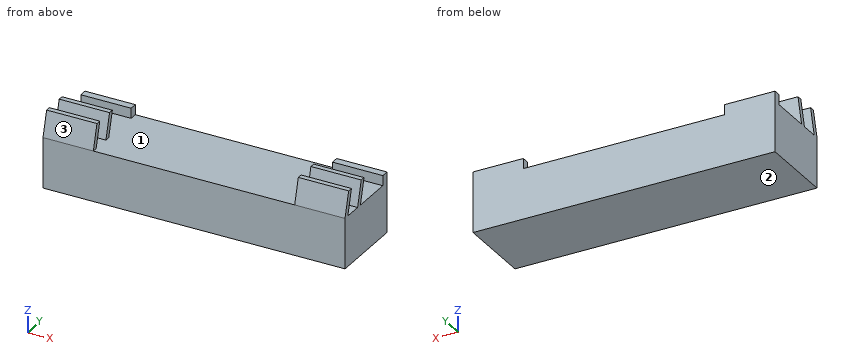
from build123d import *

# Parameters (mm, degrees)
F0_W     = 60
F0_H     = 15
F1_DEPTH = 10
F2_W     = 1.5
F2_H     = 2
F3_DEPTH = 10


with BuildPart() as f1:
    # F0 (on Top) → F1 (new body)
    with BuildSketch(Plane.XY):
        Rectangle(F0_W, F0_H)
    extrude(amount=F1_DEPTH)

    # F2 (on face) → F3 (join)
    with BuildSketch(Plane.YZ.offset(30)):
        Polygon((-6.205905, 14.829629), (-7.5, 10), (-6.5, 10), (-5.205905, 14.829629), align=None)
        Polygon((-3, 10), (-2, 10), (-0.705905, 14.829629), (-1.705905, 14.829629), align=None)
        with Locations((6.75, 11)):
            Rectangle(F2_W, F2_H)
    extrude(amount=-F3_DEPTH)

    # F4: F1 across plane


with BuildPart() as f1_1:
    add(f1.part)
    add(f1.part.mirror(Plane.YZ))


solid = f1_1.part
The model under review builds one solid part; all positions refer to its coordinate system, in mm. Face numbers are marked on the shaded views. Round coordinates to 2 decimals unless told otherwise and drop trailing zeros. Loops run counter-clockwise (first coordinate to the right, second up) from the corner with the lowest first, then second, coordinate; pieces in that order, holes last. Notation, with made-up numbers: (-19.5, 64) -> (10.5, 64) arc R18 cw to (10.5, 73) -> close; hole circle Ø9 at (9.25, 88). An arc over 180 degrees is marked (long way). Return JSON: item names as keys, results as strings.
(1) Add section B-B on x = -22. Write out the cut boundary in (y, z), plus the area to 3 significant figures.
Solved:
{"outline": "(-7.5, 0) -> (7.5, 0) -> (7.5, 12) -> (6, 12) -> (6, 10) -> (-2, 10) -> (-0.71, 14.83) -> (-1.71, 14.83) -> (-3, 10) -> (-6.5, 10) -> (-5.21, 14.83) -> (-6.21, 14.83) -> (-7.5, 10) -> close", "area": "163 mm2"}
(2) Add section C-C on z = 13.5. Write out the cut boundary in (x, y).
Solved:
{"outline": "(-30, -6.56) -> (-20, -6.56) -> (-20, -5.56) -> (-30, -5.56) -> close; (-30, -2.06) -> (-20, -2.06) -> (-20, -1.06) -> (-30, -1.06) -> close; (20, -6.56) -> (30, -6.56) -> (30, -5.56) -> (20, -5.56) -> close; (20, -2.06) -> (30, -2.06) -> (30, -1.06) -> (20, -1.06) -> close"}
(3) For pin 1 (2 mm diameter, centred on x = 15.5, y = -5, fed in from +Z); pin 2 (1.6 mm diameter, centred on x = 26, z = 11, fed in from -Y); pin 3 (1.6 mm diameter, centred on x = -23, y = 7, fed in from +Z); pin 4 (1.1 mm diameter, centred on y = -7, z = 12, fed in from +X), all flat-tipped, find the tip position at first contact; note any pin that passes through.
Solved:
{"pin 1": "z = 10", "pin 2": "y = -7.45", "pin 3": "z = 12", "pin 4": "x = 30"}
(4) Add section A-A on z = 10.75. Write out the cut boundary in (x, y).
Solved:
{"outline": "(-30, -7.3) -> (-20, -7.3) -> (-20, -6.3) -> (-30, -6.3) -> close; (-30, -2.8) -> (-20, -2.8) -> (-20, -1.8) -> (-30, -1.8) -> close; (-30, 6) -> (-20, 6) -> (-20, 7.5) -> (-30, 7.5) -> close; (20, -7.3) -> (30, -7.3) -> (30, -6.3) -> (20, -6.3) -> close; (20, -2.8) -> (30, -2.8) -> (30, -1.8) -> (20, -1.8) -> close; (20, 6) -> (30, 6) -> (30, 7.5) -> (20, 7.5) -> close"}
(5) The part is to be moulded in two halves that separate along Y. For the marked faces 1, 2 and 3, say which applies: released by +Y, released by -Y, zero draft, split by the parting line, or undercut.
Solved:
{"face 1": "undercut", "face 2": "zero draft", "face 3": "released by -Y"}
(6) For line 1 (Y direction, x = -25, z = 11); line 2 (X direction, y = -2.5, z = 11.75); line 3 (Z direction, x = 12, y = 2), list the stretches that pass through material, from the lowest coordinate up.
Solved:
{"line 1": "-7.23 to -6.23, -2.73 to -1.73, 6 to 7.5", "line 2": "-30 to -20, 20 to 30", "line 3": "0 to 10"}
(7) Add section D-D on y = -3.75. Write out the cut boundary in (x, z).
Solved:
{"outline": "(-30, 0) -> (30, 0) -> (30, 10) -> (-30, 10) -> close"}
